Geometry: final body of the model. Coordinates: model frame, mm. Face numbers are marked on the shaded views. A direction names the side the tool comes from. Give positions to 0.01 mm unless a question says otherwise; leave off trailing zeros. Write each loop counter-clockwise with the first axis right and the second up, starting at its lowest first coordinate (ties: lowest second). Pieces come first, ordered by that corner, then holes. Notation, with made-up numbers: M 35,-30.5 L 51,-30.5 A18 ccw 51,4.5 Z; hole C -27,83.25 d7. An arc over 180 degrees is marked long. Use a Markdown table: item, result. Add a question column.
(1) Cut plane A-A (z = 12). Output: boundary loops of the cut face in (x, y).
(2) Material intervals for L1, parallel to X at y = 59, z = 20; L2, parallel to Z at x = -1, y = 51; L3, parallel to Y at x = 3.25, z = 12, sorted ascending.
(3) Cut plane B-B (y = 59.5). Output: boundary loops of the cut face in (x, z) (3 decimals).
(4) Cut plane C-C (y = 20). Output: boundary loops of the cut face in (x, z) (3 decimals).
(5) Reachability of the marked faces 1 and 2 from +Z, -Z, +X, -X, +Y, -Y: full face, straight path, thin tool, end or side. Return the list, or none.
(6) Pin query (flat end, axial travel): pin 1 Ø5 at (x, z) = (-0.73, 20.17) entering from -Y; pin 2 Ø5 at (x, y) = (0, 27) entering from +Z. Return the tip coordinate at first contact, or that it passes through.
Autodesk Inventor part; units mm, degrees
ref_plane "YZ Plane" through (0, 0, 0) normal (1, 0, 0) x (0, 1, 0)
ref_plane "XZ Plane" through (0, 0, 0) normal (0, 1, 0) x (-1, 0, 0)
ref_plane "XY Plane" through (0, 0, 0) normal (0, 0, 1) x (1, 0, 0)
sketch "Sketch1" plane through (0, 0, 0) normal (0, 1, 0) x (-1, 0, 0)
  line L0 (-6.8943, 36.0441) -> (-6.8943, -70.6359)
  line L1 (8.3457, -70.6359) -> (8.3457, 36.0441)
  arc A0 (8.3457, 36.0441) -> (-6.8943, 36.0441) centre (0.7257, 36.0441) ccw
  arc A1 (-6.8943, -70.6359) -> (8.3457, -70.6359) centre (0.7257, -70.6359) ccw
  point P0 (0, 0)
  dimension "d2" = 15.24
  dimension "d4" = 7.62
  dimension "d5" = 15.24
  dimension "d6" = 7.62
  dimension "d8" = 106.68
  dimension "d9" = 15.24
extrude "Extrusion1" add sketch "Sketch1" along normal blind 64.77
sketch "Sketch2" plane through (0, 64.77, 0) normal (0, 1, 0) x (1, 0, 0)
  line L0 (6.8943, -36.0441) -> (6.8943, 70.6359)
  arc A0 (-8.3457, -36.0441) -> (6.8943, -36.0441) centre (-0.7257, -36.0441) ccw
  point P0 (0, 0)
  point P1 (-0.7257, -39.2191)
  point P2 (-0.7257, -29.6941)
  point P3 (-0.7257, -20.1691)
  dimension "d16" = 7.62
  dimension "d47" = 0
  dimension "d48" = 0
  dimension "d49" = 6.35
  dimension "d50" = 9.525
  dimension "d51" = 9.525
hole "Hole1" at (-0.7257, 64.77, 39.2191) at (-0.7257, 64.77, 29.6941) at (-0.7257, 64.77, 20.1691) direction (0, -1, 0) diameter 3.2766 end through all
sketch "Sketch3" plane through (0, 64.77, 0) normal (0, 1, 0) x (1, 0, 0)
  line L0 (-8.3457, 70.6359) -> (-8.3457, -36.0441)
  arc A0 (6.8943, 70.6359) -> (-8.3457, 70.6359) centre (-0.7257, 70.6359) ccw
  point P0 (0, 0)
  point P1 (-0.7257, 73.8109)
  dimension "d25" = 7.62
  dimension "d43" = 3.175
hole "Hole2" at (-0.7257, 64.77, -73.8109) direction (0, -1, 0) diameter 3.81 end through all
sketch "Sketch4" plane through (0, 64.77, 0) normal (0, 1, 0) x (1, 0, 0)
  line L0 (39.3169, 103.6547) -> (4.1003, 103.6547)
  line L1 (4.1003, 103.6547) -> (4.1003, -56.0742)
  line L2 (4.1003, -56.0742) -> (39.3169, -56.0742)
  line L3 (39.3169, -56.0742) -> (39.3169, 103.6547)
  line L4 (-5.5517, 100.2529) -> (-25.9242, 100.2529)
  line L5 (-25.9242, 100.2529) -> (-25.9242, -57.002)
  line L6 (-25.9242, -57.002) -> (-5.5517, -57.002)
  line L7 (-5.5517, -57.002) -> (-5.5517, 100.2529)
  line L8 (-8.3457, 70.6359) -> (-8.3457, -36.0441)
  line L9 (6.8943, -36.0441) -> (6.8943, 70.6359)
  point P0 (0, 0)
  dimension "d34" = 2.794
  dimension "d35" = 2.794
extrude "Extrusion2" cut sketch "Sketch4" against normal blind 101.6
sketch "Sketch5" plane through (4.1003, 64.77, 41.941) normal (1, 0, 0) x (0, 0, -1)
  line L0 (-34.9815, -12.7) -> (40.64, -12.7)
  line L1 (40.64, -12.7) -> (40.64, -52.07)
  line L2 (40.64, -52.07) -> (-34.9815, -52.07)
  line L3 (-34.9815, -52.07) -> (-34.9815, -12.7)
  line L4 (0, -64.77) -> (0, 0)
  line L5 (0, 0) -> (118.4739, 0)
  line L6 (118.4739, -64.77) -> (0, -64.77)
  point P0 (41.941, -64.77)
  dimension "d38" = 40.64
  dimension "d39" = 12.7
  dimension "d40" = 12.7
extrude "Extrusion3" cut sketch "Sketch5" against normal blind 25.4
sketch "Sketch6" plane through (0, 64.77, 0) normal (0, 1, 0) x (1, 0, 0)
  circle A0 centre (-0.7257, -29.6941) radius 1.6383
  circle A1 centre (-0.7257, -29.6941) radius 3.175
  point P0 (0, 0)
  dimension "d44" = 6.35
extrude "Extrusion4" cut sketch "Sketch6" against normal blind 101.6
properties part number "GripperArm"
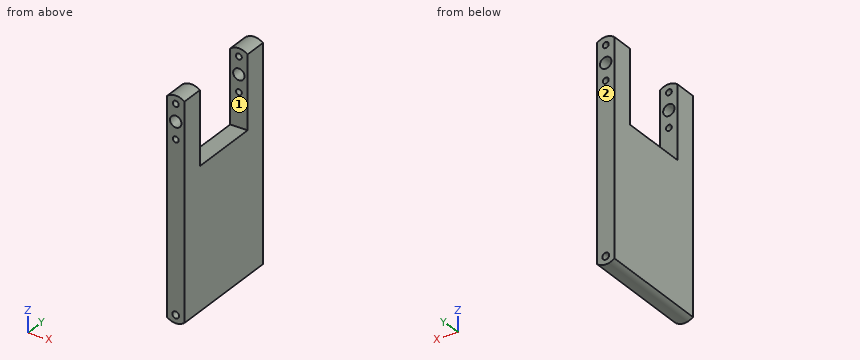
Answer list:
| question | item | result |
|---|---|---|
| 1 | outline | M -5.55,0 L 4.1,0 L 4.1,12.7 L -5.55,12.7 Z; M -5.55,52.07 L 4.1,52.07 L 4.1,64.77 L -5.55,64.77 Z |
| 2 | L1 | -5.55 to -2.36, 0.9 to 4.1 |
| 2 | L2 | -78.25 to -75.7, -71.93 to 1.3 |
| 2 | L3 | 0 to 12.7, 52.07 to 64.77 |
| 3 | outline | M -5.552,-76.533 A7.62 ccw 4.1,-76.533 L 4.1,41.941 A7.62 ccw -5.552,41.941 Z; hole C -0.726,29.694 d6.35; hole C -0.726,-73.811 d3.81; hole C -0.726,20.169 d3.277; hole C -0.726,39.219 d3.277 |
| 4 | outline | M -5.552,-76.533 A7.62 ccw 4.1,-76.533 L 4.1,1.301 L -5.552,1.301 Z; hole C -0.726,-73.811 d3.81 |
| 5 | face 1 | +Z, +X, -X |
| 5 | face 2 | +Z, -Z, +X, -X, +Y |
| 6 | pin 1 | y = 0 |
| 6 | pin 2 | z = 1.3 |
